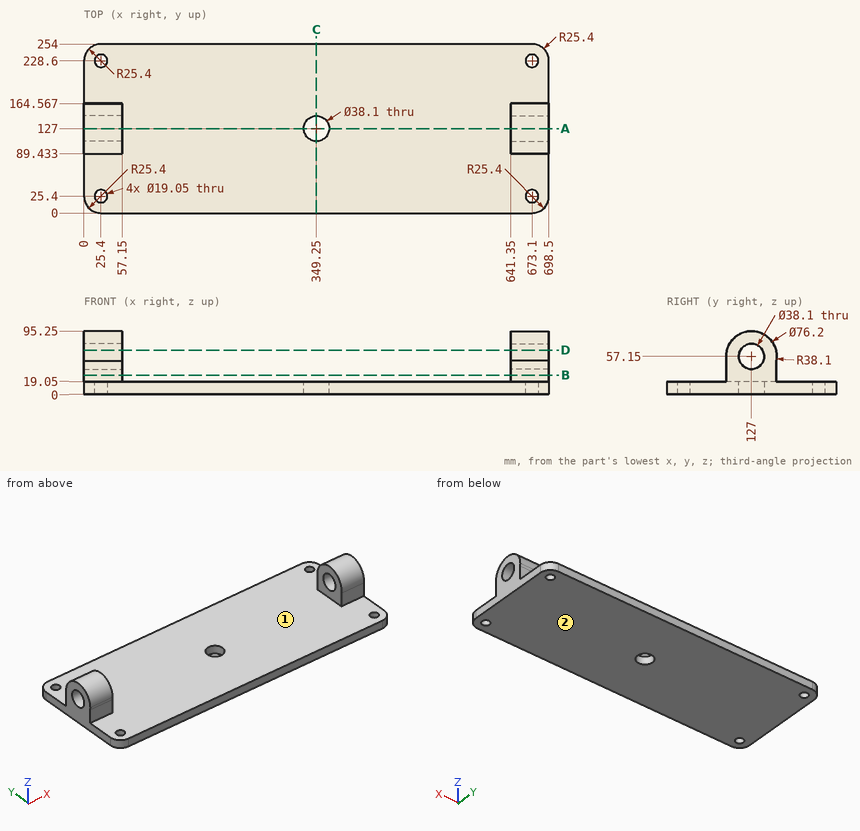
Print and shaded views of the part. All mm, measured from the part's lowest x, y and z. Coordinates: 2 decimals unless noted, no trailing zeros. Order: outer loops, then holes, each group sorted by start corner. A loop starts at its lowest first (then second) coordinate and runs counter-clockwise, first axis right, second up.
Item 1: Saw through at D-D on z = 66.5. State how many separate pieces and enclosed holes the cut face has, then the cut area to 3 significant figures.
Filled in:
separate pieces: 4
enclosed holes: 0
area: 4,650 mm2
Item 2: Drop flat-ended pins along their axis: pin 1 Ø16 at (x, z) = (23, 41) entering from +Y; pin 2 Ø25 at (x, y) = (25.4, 25.4) entering from +Z. Give the stop position or say it passes through.
Filled in:
pin 1: stops at y = 164.57
pin 2: stops at z = 19.05
Item 3: Saw through at C-C on x = 349.25. List the corners of the cut face in (y, z), then the cut area to 3 significant figures.
Filled in:
outline: (0, 0) - (107.95, 0) - (107.95, 19.05) - (0, 19.05) - close; (146.05, 0) - (254, 0) - (254, 19.05) - (146.05, 19.05) - close
area: 4,110 mm2
Item 4: Saw through at A-A on y = 127. List the corners of the cut face in (x, z).
Filled in:
outline: (0, 0) - (330.2, 0) - (330.2, 19.05) - (57.15, 19.05) - (57.15, 38.1) - (0, 38.1) - close; (0, 76.2) - (57.15, 76.2) - (57.15, 95.25) - (0, 95.25) - close; (368.3, 0) - (698.5, 0) - (698.5, 38.1) - (641.35, 38.1) - (641.35, 19.05) - (368.3, 19.05) - close; (641.35, 76.2) - (698.5, 76.2) - (698.5, 95.25) - (641.35, 95.25) - close
Item 5: Drill centre lines: L1, parallel to Y at x = 673.1, z = 10.5 (3 decimals); L2, parallel to X at y = 127, z = 12.75; L3, parallel to X at y = 132.5, z = 89. Where is each one in solid material? Low to high.
Filled in:
L1: y = 0 to 15.875, 34.925 to 219.075, 238.125 to 254
L2: x = 0 to 330.2, 368.3 to 698.5
L3: x = 0 to 57.15, 641.35 to 698.5
Item 6: Saw through at B-B on z = 29. List the corners of the cut face in (x, y).
Filled in:
outline: (0, 89.43) - (57.15, 89.43) - (57.15, 164.57) - (0, 164.57) - close; (641.35, 89.43) - (698.5, 89.43) - (698.5, 164.57) - (641.35, 164.57) - close
Item 7: Mould opens along X. For the marked faces 1 and 2 say: released by +X, released by -X, zero draft, split by the parting line, or undercut.
Filled in:
face 1: undercut
face 2: zero draft
